Job drawing, mm, ordinate dimensions from the low corner. One solid piece. A direction names the side the tool comes from. Coordinates: 2 decimals unless noted, no trailing zeros. Loops run counter-clockwise (first coordinate to the right, second up) from the corner with the lowest first, then second, coordinate; pieces in that order, holes last. Notation, with made-up numbers: (58, 67) - (110, 67) arc R12 ccw to (110, 73) - close; hole circle Ø8 at (85, -4.75). An arc over 180 degrees is marked (long way). Use a Markdown table: item, result. Add a question column.
1) Band-saw the part on D-D (x = 46). Give the cut face in (y, z), plus the area to 3 significant figures.
2) Band-saw the part on B-B (z = 5). Give the cut face in (x, y), plus the area to 3 significant figures.
3) Band-saw the part on A-A (z = 20.5). Give the cut face in (x, y).
4) Band-saw the part on C-C (x = 19). Give the cut face in (y, z), plus the area to 3 significant figures.
5) Tool access for the marked faces 1 and 2: list every direction of +Z, -Z, +X, -X, +Y, -Y with a clear straight run to the whole face (end or side of a thin tool).
6) Probe probe 1 along Z at (x, y) = (15, 56.85); probe 2 along Y at (x, z) = (19.5, 7.5); probe 3 along X at (y, z) = (8, 10). List the from-to ranges inside material, lowest first. Write a range as [from, to].
7) Drop a flat-ended pin along its axis: P1, Ø3, axis at x = 15, z = 36, coming from the -Y side. Give the stop position or say it passes through.
8) Pull direction Y, two halves, no side cores. Call the marked faces 3, 4, 5 and 6: +Y half, -Y half, draft (parallel to the pull), parting line (faces both ways), or undercut.
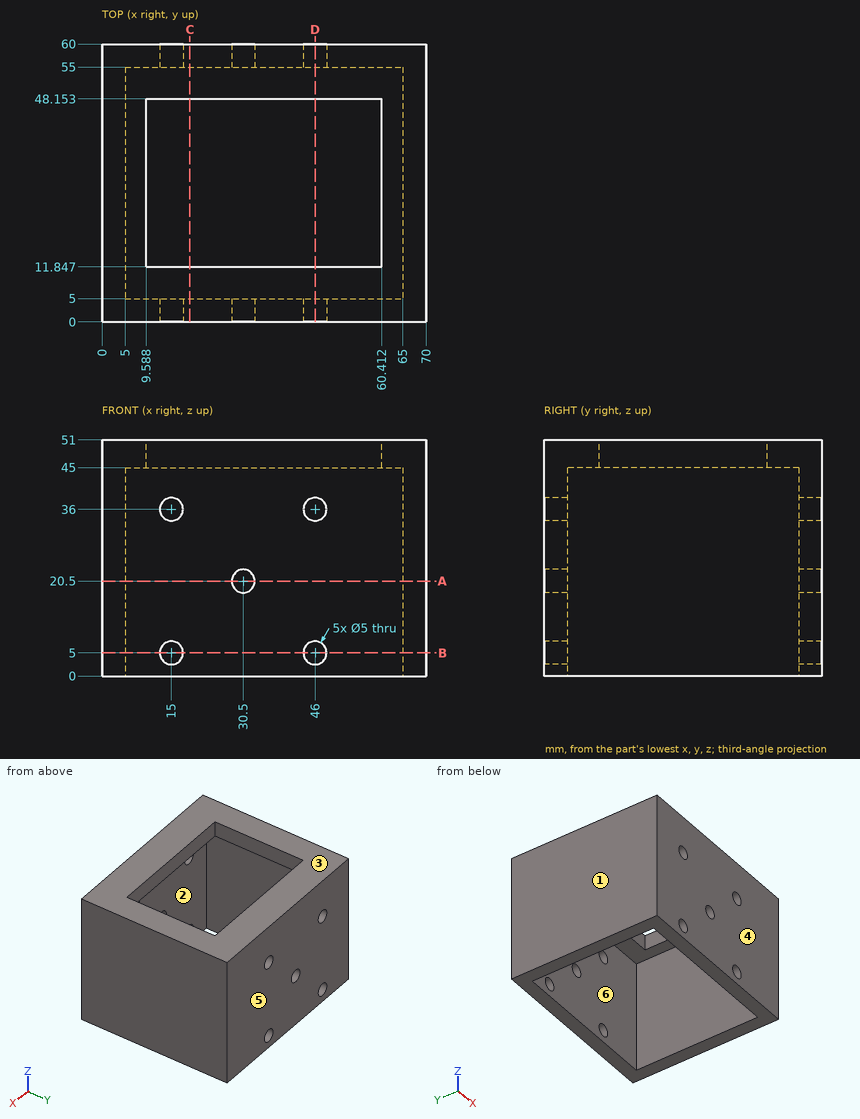
Answer block:
| question | item | result |
|---|---|---|
| 1 | outline | (0, 0) - (5, 0) - (5, 2.5) - (0, 2.5) - close; (0, 7.5) - (5, 7.5) - (5, 33.5) - (0, 33.5) - close; (0, 38.5) - (5, 38.5) - (5, 45) - (11.85, 45) - (11.85, 51) - (0, 51) - close; (48.15, 45) - (55, 45) - (55, 38.5) - (60, 38.5) - (60, 51) - (48.15, 51) - close; (55, 0) - (60, 0) - (60, 2.5) - (55, 2.5) - close; (55, 7.5) - (60, 7.5) - (60, 33.5) - (55, 33.5) - close |
| 1 | area | 492 mm2 |
| 2 | outline | (0, 0) - (12.5, 0) - (12.5, 5) - (5, 5) - (5, 55) - (12.5, 55) - (12.5, 60) - (0, 60) - close; (17.5, 0) - (43.5, 0) - (43.5, 5) - (17.5, 5) - close; (17.5, 55) - (43.5, 55) - (43.5, 60) - (17.5, 60) - close; (48.5, 0) - (70, 0) - (70, 60) - (48.5, 60) - (48.5, 55) - (65, 55) - (65, 5) - (48.5, 5) - close |
| 2 | area | 1,100 mm2 |
| 3 | outline | (0, 0) - (28, 0) - (28, 5) - (5, 5) - (5, 55) - (28, 55) - (28, 60) - (0, 60) - close; (33, 0) - (70, 0) - (70, 60) - (33, 60) - (33, 55) - (65, 55) - (65, 5) - (33, 5) - close |
| 4 | outline | (0, 0) - (5, 0) - (5, 45) - (11.85, 45) - (11.85, 51) - (0, 51) - close; (48.15, 45) - (55, 45) - (55, 0) - (60, 0) - (60, 51) - (48.15, 51) - close |
| 4 | area | 592 mm2 |
| 5 | face 1 | +Z, -Z, -X, +Y, -Y |
| 5 | face 2 | -Z |
| 6 | probe 1 | [0, 2.5], [7.5, 33.5], [38.5, 51] |
| 6 | probe 2 | [0, 5], [55, 60] |
| 6 | probe 3 | [0, 5], [65, 70] |
| 7 | P1 | through |
| 8 | face 3 | draft |
| 8 | face 4 | -Y half |
| 8 | face 5 | +Y half |
| 8 | face 6 | undercut |
